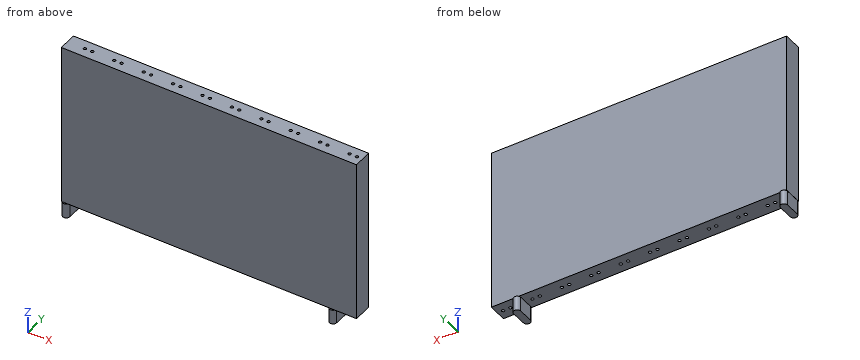
from build123d import *

# Parameters (mm, degrees)
SKETCH_W     = 101.9675
SKETCH_H     = 6.5
PAD_DEPTH    = 56.05
SKETCH001_R  = 0.5
POCKET_DEPTH = 70
PAD001_DEPTH = 5


with BuildPart() as part:
    # Sketch → Pad (new body)
    with BuildSketch(Plane.XY):
        with Locations((-2.03875, 0)):
            Rectangle(SKETCH_W, SKETCH_H)
    extrude(amount=PAD_DEPTH)

    # Sketch001 (on Face6 of Pad) → Pocket (cut)
    with BuildSketch(Plane.XY.offset(56.05)):
        with Locations((3.81, 0)):
            Circle(SKETCH001_R)
        with Locations((6.35, 0)):
            Circle(SKETCH001_R)
        with Locations((-16.51, 0)):
            Circle(SKETCH001_R)
        with Locations((-13.97, 0)):
            Circle(SKETCH001_R)
        with Locations((-34.29, 0)):
            Circle(SKETCH001_R)
        with Locations((-36.83, 0)):
            Circle(SKETCH001_R)
        with Locations((13.97, 0)):
            Circle(SKETCH001_R)
        with Locations((16.51, 0)):
            Circle(SKETCH001_R)
        with Locations((24.13, 0)):
            Circle(SKETCH001_R)
        with Locations((26.67, 0)):
            Circle(SKETCH001_R)
        with Locations((34.29, 0)):
            Circle(SKETCH001_R)
        with Locations((36.83, 0)):
            Circle(SKETCH001_R)
        with Locations((44.45, 0)):
            Circle(SKETCH001_R)
        with Locations((46.99, 0)):
            Circle(SKETCH001_R)
        with Locations((-46.99, 0)):
            Circle(SKETCH001_R)
        with Locations((-44.45, 0)):
            Circle(SKETCH001_R)
        with Locations((-26.67, 0)):
            Circle(SKETCH001_R)
        with Locations((-24.13, 0)):
            Circle(SKETCH001_R)
        with Locations((-6.35, 0)):
            Circle(SKETCH001_R)
        with Locations((-3.81, 0)):
            Circle(SKETCH001_R)
    extrude(amount=-POCKET_DEPTH, mode=Mode.SUBTRACT)

    # Sketch002 (on Face4 of Pocket) → Pad001 (join)
    with BuildSketch(Plane(origin=(0, 0, 0), x_dir=(1, 0, 0), z_dir=(0, 0, -1))):
        with BuildLine():
            Line((-50.52, 2.56), (-50.52, -2.56))
            ThreePointArc((-52.97, -2.56), (-51.745, -3.789911), (-50.52, -2.56))
            Line((-52.97, -2.56), (-52.97, 2.56))
            ThreePointArc((-50.52, 2.56), (-51.745, 3.795206), (-52.97, 2.56))
        make_face()
        with BuildLine():
            Line((41.66, 2.56), (41.66, -2.56))
            ThreePointArc((39.21, -2.56), (40.435, -3.757758), (41.66, -2.56))
            Line((39.21, -2.56), (39.21, 2.56))
            ThreePointArc((41.66, 2.56), (40.435, 3.795415), (39.21, 2.56))
        make_face()
    extrude(amount=PAD001_DEPTH)


solid = part.part
CAD build for the part. Positions are in the model's coordinates, mm. Give positions to 0.01 mm unless a question says otherwise; leave off trailing zeros. Write each loop counter-clockwise with the first axis right and the second up, starting at its lowest first coordinate (ties: lowest second). Pieces come first, ordered by that corner, then holes. Notation, with made-up numbers: M 61.25,81.5 L 117.25,81.5 A22 ccw 117.25,103.5 Z; hole C -1,39.5 d7. An arc over 180 degrees is marked long. Put each result on its own line as item: value. Start each with the question number.
(1) Flat gauge pins, fed straight in: pin 1 Ø17 at (x, z) = (23.5, 19.5) entering from -Y; pin 2 Ø2.5 at (y, z) = (0.5, -3) entering from -X; pin 3 Ø2.5 at (y, z) = (-0.5, -2.5) entering from +X. Where does each tip first touch, or does it go through?
(2) Probe L1, parallel to X at y = 1.5, z = -0.5; L2, parallel to Y at x = 6.5, z = 13; L3, parallel to Z at x = 37, y = 1.25. List the from-to ranges inside material, lowest first.
(3) Band-saw the part on A-A, the plane z = 21.5. Give the number of separate pieces and of enclosed holes in the cut face, and give its area (3 significant figures).
(4) Band-saw the part on B-B, the plane x = -29. Write the cut outline in (y, z).
Response values:
1. pin 1: stops at y = -3.25
1. pin 2: stops at x = -52.97
1. pin 3: stops at x = 41.66
2. L1: x = -52.97 to -50.52, 39.21 to 41.66
2. L2: y = -3.25 to -0.48, 0.48 to 3.25
2. L3: z = 0 to 56.05
3. separate pieces: 1
3. enclosed holes: 20
3. area: 647 mm2
4. outline: M -3.25,0 L 3.25,0 L 3.25,56.05 L -3.25,56.05 Z
